The listing builds one solid part. Answer for the finished solid, in the listing's coordinates (mm). A direction names the side the tool comes from. Coordinates: 2 decimals unless noted, no trailing zeros. Order: outer loops, then holes, each group sorted by start corner. A loop starts at its lowest first (then second) coordinate and runs counter-clockwise, first axis right, second up. Notation, with made-up numbers: M 37,-9 L 79,-9 A19 ccw 79,24 Z; hole C 80.5,-30.75 d10. An arc over 180 degrees is marked long. One line per item, written item: value. Start each with the question number.
Q1. The part is cut by section A-A on x = 0. Give the vertices of the cut face in (y, z), then the cut area to 3 significant figures.
Q2. Each of these flat-tipped pins is pushed along its axis until it touches: pin 1 Ø1 at (y, z) = (2, 12.5) entering from -X; pin 2 Ø2 at (x, z) = (0.5, 6) entering from +Y; pin 3 Ø0.7 at (x, y) = (0.5, 3.5) entering from +Z. Where does it stop, or does it pass through?
Q3. The part is cut by section D-D on z = 12. Give the vertices of the cut face in (x, y), then the cut area to 3 significant figures.
Q4. The part is cut by section C-C on y = 3.25. Give the vertices of the cut face in (x, z).
Q5. Determine the mould class of faces 4 (the cylindrical face through (2.262, -1.734, 2.197)), 5 (the flat face through (0, 4, 15.4)), 6 (the cylindrical face through (-3, 0, 1)), 7 (the cylindrical face through (0.62, 2.78, 24.6)) for opening direction Z: pulls with the +Z half, pulls with the -Z half, needs draft (parallel to the pull), parting line crosses it, or undercut.
Q6. Straight lines are drawn through the part: line 1 along Z through (x, y) = (2.65, 0.75); line 2 along Y through (x, z) = (1.2, 18.75); line 3 along Y through (x, z) = (0.05, 16.75). For each, find the intervals that lie inside material, in ascending order. Write a range as [from, to].
Q7. For faces 1 (the flat face through (-0.9, 4, 13)), 2 (the flat face through (0.9, 4, 13)), 3 (the flat face through (0, 0, 26.8)), determine the directions among +Z, -Z, +X, -X, +Y, -Y from which every point of the face is accessible in a straight line to the end or side of a thin tool.
Q8. The part is cut by section B-B on z = 8.5. Give the vertices of the cut face in (x, y).
```python
from build123d import *

# Parameters (mm, degrees)
SKETCH1_R           = 3
BOSS_EXTRUDE1_DEPTH = 26.8
BOSS_EXTRUDE2_START = -11.4
SKETCH2_W           = 1.8
SKETCH2_H           = 4.2
BOSS_EXTRUDE2_DEPTH = 4
CUT_EXTRUDE1_START  = -2
SKETCH3_R           = 3
SKETCH3_R_2         = 2.85
CUT_EXTRUDE1_DEPTH  = 0.4
CUT_EXTRUDE2_START  = -2.4
SKETCH4_R           = 3.000966843
SKETCH4_R_2         = 2.85
CUT_EXTRUDE2_DEPTH  = 0.4
CHAMFER1_SIZE       = 0.25


with BuildPart() as part:
    # Sketch1 → Boss-Extrude1 (new body)
    with BuildSketch(Plane.XY):
        Circle(SKETCH1_R)
    extrude(amount=BOSS_EXTRUDE1_DEPTH)

    # Sketch2 → Boss-Extrude2 (add)
    with BuildSketch(Plane(origin=(0, 0, 0), x_dir=(-1, 0, 0), z_dir=(0, 0, -1)).offset(BOSS_EXTRUDE2_START)):
        with Locations((0, 2.1)):
            Rectangle(SKETCH2_W, SKETCH2_H)
    extrude(amount=-BOSS_EXTRUDE2_DEPTH)

    # Sketch3 → Cut-Extrude1 (cut)
    with BuildSketch(Plane(origin=(0, 0, 0), x_dir=(-1, 0, 0), z_dir=(0, 0, -1)).offset(CUT_EXTRUDE1_START)):
        Circle(SKETCH3_R)
        Circle(SKETCH3_R_2, mode=Mode.SUBTRACT)
    extrude(amount=-CUT_EXTRUDE1_DEPTH, mode=Mode.SUBTRACT)

    # Sketch4 → Cut-Extrude2 (cut)
    with BuildSketch(Plane.XY.offset(26.8).offset(CUT_EXTRUDE2_START)):
        Circle(SKETCH4_R)
        with Locations(Location((0, 0, 0), (0, 0, 180))):
            Circle(SKETCH4_R_2, mode=Mode.SUBTRACT)
    extrude(amount=CUT_EXTRUDE2_DEPTH, mode=Mode.SUBTRACT)

    # Chamfer1
    chamfer1_edges = [part.edges().sort_by_distance(p)[0] for p in [
        (-3, 0, 0),
        (-3, 0, 26.8),
    ]]
    chamfer(chamfer1_edges, length=CHAMFER1_SIZE)


solid = part.part
```
Output:
1. outline: M -3,0.25 L -2.75,0 L 2.75,0 L 3,0.25 L 3,2 L 2.85,2 L 2.85,2.4 L 3,2.4 L 3,11.4 L 4.2,11.4 L 4.2,15.4 L 3,15.4 L 3,24.4 L 2.85,24.4 L 2.85,24.8 L 3,24.8 L 3,26.55 L 2.75,26.8 L -2.75,26.8 L -3,26.55 L -3,24.8 L -2.85,24.8 L -2.85,24.4 L -3,24.4 L -3,2.4 L -2.85,2.4 L -2.85,2 L -3,2 Z
1. area: 165 mm^2
2. pin 1: stops at x = -2.6
2. pin 2: stops at y = 3
2. pin 3: stops at z = 15.4
3. outline: M -0.9,2.86 A3 ccw long 0.9,2.86 L 0.9,4.2 L -0.9,4.2 Z
3. area: 30.5 mm^2
4. outline: M -0.9,11.4 L 0.9,11.4 L 0.9,15.4 L -0.9,15.4 Z
5. face 4: undercut
5. face 5: pulls with the +Z half
5. face 6: needs draft
5. face 7: undercut
6. line 1: z = [0, 26.8]
6. line 2: y = [-2.75, 2.75]
6. line 3: y = [-3, 3]
7. face 1: +Z, -Z, -X, +Y
7. face 2: +Z, -Z, +X, +Y
7. face 3: +Z, +X, -X, +Y, -Y
8. outline: C 0,0 d6
